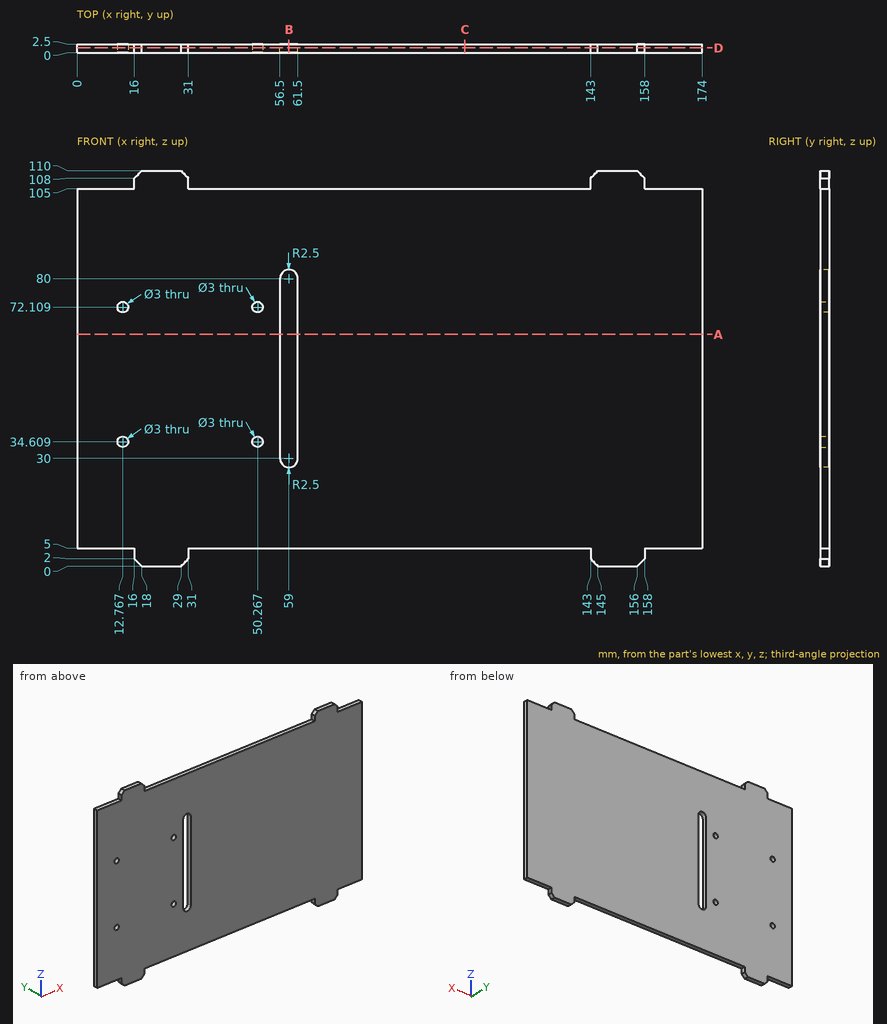
Answer from the drawing. Dimensions are ordinates in mm from the lowest x, y and z of the part. Coordinates: 2 decimals unless noted, no trailing zeros. Write each loop counter-clockwise with the first axis right and the second up, starting at its lowest first coordinate (ties: lowest second). Pieces come first, ordered by that corner, then holes. Notation, with made-up numbers: M -7,6 L -1,6 A14 ccw -1,18 Z; hole C 41.5,28.25 d10. An arc over 180 degrees is marked long. Write item = value, one per line.
1. Straight lines are drawn through the part: line 1 (X direction, y = 1.6, z = 39); line 2 (Z direction, x = 49.5, y = 1.7); line 3 (Z direction, x = 158.5, y = 2.15). For each, find the intervals that lie inside material, in ascending order. Write a range as from..to.
Solution:
line_1 = 0..56.5, 61.5..174
line_2 = 5..33.32, 35.9..70.82, 73.4..105
line_3 = 5..105
2. The part is cut by section C-C (x = 108). Determine the outline of the cut face in (y, z), then the cut area to 3 significant figures.
Solution:
outline = M 0,5 L 2.5,5 L 2.5,105 L 0,105 Z
area = 250 mm2
3. The part is cut by section A-A (z = 64.5). Determine the outline of the cut face in (x, y).
Solution:
outline = M 0,0 L 56.5,0 L 56.5,2.5 L 0,2.5 Z; M 61.5,0 L 174,0 L 174,2.5 L 61.5,2.5 Z
4. The part is cut by section D-D (y = 1.45). State how many separate pieces and enclosed holes the cut face has, then the cut area to 3 significant figures.
Solution:
separate_pieces = 1
enclosed_holes = 5
area = 17,400 mm2
5. Flat-ended cylindrical pins translate along their axes: pin 1 (0.8 mm diameter, centred on x = 88.5, y = 1.5, fed in from +Z); pin 2 (1.2 mm diameter, centred on x = 9, y = 0.5, fed in from -Z); pin 3 (1.2 mm diameter, centred on y = 1.5, z = 106, fed in from +X). Find the tip coordinate at first contact, or state that the pin passes through.
Solution:
pin_1 = 105
pin_2 = 5
pin_3 = 158
6. The part is cut by section B-B (x = 59). Determine the outline of the cut face in (y, z).
Solution:
outline = M 0,5 L 2.5,5 L 2.5,27.5 L 0,27.5 Z; M 0,82.5 L 2.5,82.5 L 2.5,105 L 0,105 Z
